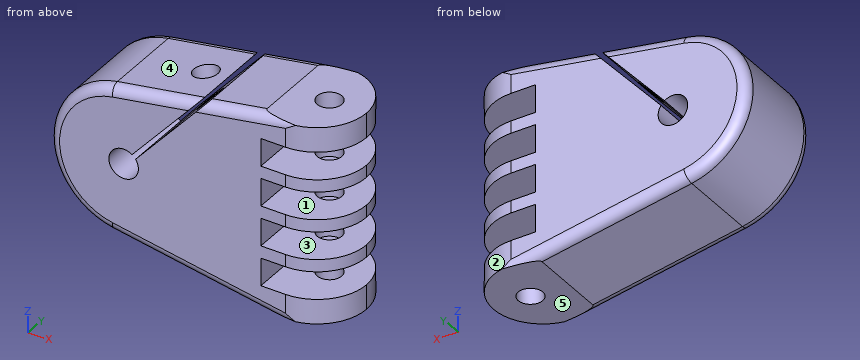
from build123d import *

# Parameters (mm, degrees)
BOSS_EXTRUDE1_DEPTH = 20
FILLET1_R           = 10
SKETCH2_R           = 2.5
CUT_EXTRUDE1_DEPTH  = 40
FILLET2_R           = 2
SKETCH3_R           = 2.5
CUT_EXTRUDE2_DEPTH  = 10
SKETCH4_R           = 10
SKETCH4_R_2         = 3
BOSS_EXTRUDE2_DEPTH = 20
CUT_EXTRUDE3_DEPTH  = 52.342938219


# Some blends are built 0.0001 mm under size
with BuildPart() as part:
    # Sketch1 → Boss-Extrude1 (new body)
    with BuildSketch(Plane(origin=(0, 0, 0), x_dir=(1, 0, 0), z_dir=(0, 1, 0))):
        with BuildLine():
            Line((27.849705815, 9.375), (27.849705815, 15))
            Line((27.849705815, 15), (42.849705815, 15))
            Line((42.849705815, 15), (42.849705815, 20))
            Line((42.849705815, 20), (27.849705815, 20))
            Line((27.849705815, 20), (-2.537743238, 14.78377013))
            ThreePointArc((-2.537743238, 14.78377013), (-15, 0), (-2.537743238, -14.78377013))
            Line((-2.537743238, -14.78377013), (15.176440556, -17.824540498))
            Line((15.176440556, -17.824540498), (6.327966589, -7.743180151))
            ThreePointArc((6.327966589, -7.743180151), (-6.707251498, 7.417059885), (7.069754095, -7.072381285))
            Line((7.069754095, -7.072381285), (16.743020962, -18.093455585))
            Line((16.743020962, -18.093455585), (27.849705815, -20))
            Line((27.849705815, -20), (42.849705815, -20))
            Line((42.849705815, -20), (42.849705815, -15))
            Line((42.849705815, -15), (27.849705815, -15))
            Line((27.849705815, -15), (27.849705815, -9.375))
            Line((27.849705815, -9.375), (42.849705815, -9.375))
            Line((42.849705815, -9.375), (42.849705815, -6.875))
            Line((42.849705815, -6.875), (27.849705815, -6.875))
            Line((27.849705815, -6.875), (27.849705815, -1.25))
            Line((27.849705815, -1.25), (42.849705815, -1.25))
            Line((42.849705815, -1.25), (42.849705815, 1.25))
            Line((42.849705815, 1.25), (27.849705815, 1.25))
            Line((27.849705815, 1.25), (27.849705815, 6.875))
            Line((27.849705815, 6.875), (42.849705815, 6.875))
            Line((42.849705815, 6.875), (42.849705815, 9.375))
            Line((42.849705815, 9.375), (27.849705815, 9.375))
        make_face()
    extrude(amount=BOSS_EXTRUDE1_DEPTH)

    # Fillet1
    fillet1_edges = [part.edges().sort_by_distance(p)[0] for p in [
        (42.849705815, 0, 17.5),
        (42.849705815, 0, 8.125),
        (42.849705815, 0, 0),
        (42.849705815, 0, -8.125),
        (42.849705815, 0, -17.5),
        (42.849705815, 20, -17.5),
        (42.849705815, 20, -8.125),
        (42.849705815, 20, 0),
        (42.849705815, 20, 8.125),
        (42.849705815, 20, 17.5),
    ]]
    fillet(fillet1_edges, radius=FILLET1_R - 0.0001)  # a hair under: the kernel refuses the full size

    # Sketch2 → Cut-Extrude1 (cut)
    with BuildSketch(Plane(origin=(0, 0, -20), x_dir=(-1, 0, 0), z_dir=(0, 0, -1))):
        with Locations((-35.349705815, 10)):
            Circle(SKETCH2_R)
    extrude(amount=-CUT_EXTRUDE1_DEPTH, mode=Mode.SUBTRACT)

    # Fillet2
    # the kernel refuses this fillet: 2 mm, written as the material it takes off along each edge
    with BuildSketch(Plane(origin=(39.676721919, 0, -22.03019459), x_dir=(0.16918288251037936, 0, 0.9855846753402162), z_dir=(-0.9855846753402161, 0, 0.16918288251037933))) as fillet2_piece_1:
        with BuildLine():
            CenterArc((FILLET2_R, FILLET2_R), FILLET2_R, 180, 90)
            Line((0, FILLET2_R), (-FILLET2_R * 0.02, FILLET2_R))
            Line((-FILLET2_R * 0.02, FILLET2_R), (-FILLET2_R * 0.02, -FILLET2_R * 0.02))
            Line((-FILLET2_R * 0.02, -FILLET2_R * 0.02), (FILLET2_R, -FILLET2_R * 0.02))
            Line((FILLET2_R, -FILLET2_R * 0.02), (FILLET2_R, 0))
        make_face()
    extrude(amount=42.831900914, mode=Mode.SUBTRACT)
    with BuildSketch(Plane(origin=(-2.537743238, 0, 14.78377013), x_dir=(0.16918288251037944, 0, -0.9855846753402161), z_dir=(0.9855846753402161, 0, 0.16918288251037944))) as fillet2_piece_2:
        with BuildLine():
            CenterArc((FILLET2_R, FILLET2_R), FILLET2_R, 180, 90)
            Line((0, FILLET2_R), (-FILLET2_R * 0.02, FILLET2_R))
            Line((-FILLET2_R * 0.02, FILLET2_R), (-FILLET2_R * 0.02, -FILLET2_R * 0.02))
            Line((-FILLET2_R * 0.02, -FILLET2_R * 0.02), (FILLET2_R, -FILLET2_R * 0.02))
            Line((FILLET2_R, -FILLET2_R * 0.02), (FILLET2_R, 0))
        make_face()
    extrude(amount=29.973274379, mode=Mode.SUBTRACT)
    with BuildSketch(Plane(origin=(39.676721919, 20, -22.03019459), x_dir=(0.16918288251037936, 0, 0.9855846753402162), z_dir=(-0.9855846753402161, 0, 0.16918288251037933))) as fillet2_piece_3:
        with BuildLine():
            CenterArc((FILLET2_R, -FILLET2_R), FILLET2_R, 90, 90)
            Line((0, -FILLET2_R), (-FILLET2_R * 0.02, -FILLET2_R))
            Line((-FILLET2_R * 0.02, -FILLET2_R), (-FILLET2_R * 0.02, FILLET2_R * 0.02))
            Line((-FILLET2_R * 0.02, FILLET2_R * 0.02), (FILLET2_R, FILLET2_R * 0.02))
            Line((FILLET2_R, FILLET2_R * 0.02), (FILLET2_R, 0))
        make_face()
    extrude(amount=42.831900914, mode=Mode.SUBTRACT)
    with BuildSketch(Plane(origin=(-2.537743238, 20, 14.78377013), x_dir=(0.16918288251037944, 0, -0.9855846753402161), z_dir=(0.9855846753402161, 0, 0.16918288251037944))) as fillet2_piece_4:
        with BuildLine():
            CenterArc((FILLET2_R, -FILLET2_R), FILLET2_R, 90, 90)
            Line((0, -FILLET2_R), (-FILLET2_R * 0.02, -FILLET2_R))
            Line((-FILLET2_R * 0.02, -FILLET2_R), (-FILLET2_R * 0.02, FILLET2_R * 0.02))
            Line((-FILLET2_R * 0.02, FILLET2_R * 0.02), (FILLET2_R, FILLET2_R * 0.02))
            Line((FILLET2_R, FILLET2_R * 0.02), (FILLET2_R, 0))
        make_face()
    extrude(amount=29.973274379, mode=Mode.SUBTRACT)
    with BuildSketch(Plane(origin=(4.916004858, 0, 16.063260995), x_dir=(0.16918288251037944, 0, -0.9855846753402161), z_dir=(0.9855846753402161, 0, 0.16918288251037944))) as fillet2_piece_5:
        with BuildLine():
            CenterArc((FILLET2_R, FILLET2_R), FILLET2_R, 180, 90)
            Line((0, FILLET2_R), (-FILLET2_R * 0.02, FILLET2_R))
            Line((-FILLET2_R * 0.02, FILLET2_R), (-FILLET2_R * 0.02, -FILLET2_R * 0.02))
            Line((-FILLET2_R * 0.02, -FILLET2_R * 0.02), (FILLET2_R, -FILLET2_R * 0.02))
            Line((FILLET2_R, -FILLET2_R * 0.02), (FILLET2_R, 0))
        make_face()
    extrude(amount=35.269133064, mode=Mode.SUBTRACT)
    with BuildSketch(Plane(origin=(4.916004858, 20, 16.063260995), x_dir=(0.16918288251037944, 0, -0.9855846753402161), z_dir=(0.9855846753402161, 0, 0.16918288251037944))) as fillet2_piece_6:
        with BuildLine():
            CenterArc((FILLET2_R, -FILLET2_R), FILLET2_R, 90, 90)
            Line((0, -FILLET2_R), (-FILLET2_R * 0.02, -FILLET2_R))
            Line((-FILLET2_R * 0.02, -FILLET2_R), (-FILLET2_R * 0.02, FILLET2_R * 0.02))
            Line((-FILLET2_R * 0.02, FILLET2_R * 0.02), (FILLET2_R, FILLET2_R * 0.02))
            Line((FILLET2_R, FILLET2_R * 0.02), (FILLET2_R, 0))
        make_face()
    extrude(amount=35.269133064, mode=Mode.SUBTRACT)
    with BuildSketch(Plane(origin=(0, 0, 0), x_dir=(-0.16918288251037905, 0, -0.9855846753402162), z_dir=(0.9855846753402162, 0, -0.16918288251037905))) as fillet2_piece_7:
        with BuildLine():
            CenterArc((15 - FILLET2_R, FILLET2_R), FILLET2_R, 270, 90)
            Line((15, FILLET2_R), (15 + FILLET2_R * 0.02, FILLET2_R))
            Line((15 + FILLET2_R * 0.02, FILLET2_R), (15 + FILLET2_R * 0.02, -FILLET2_R * 0.02))
            Line((15 + FILLET2_R * 0.02, -FILLET2_R * 0.02), (15 - FILLET2_R, -FILLET2_R * 0.02))
            Line((15 - FILLET2_R, -FILLET2_R * 0.02), (15 - FILLET2_R, 0))
        make_face()
    revolve(axis=Axis((0, 0, 0), (0, 1, 0)), revolution_arc=160.519372943, mode=Mode.SUBTRACT)
    with BuildSketch(Plane(origin=(0, 20, 0), x_dir=(-0.16918288251037905, 0, -0.9855846753402162), z_dir=(0.9855846753402162, 0, -0.16918288251037905))) as fillet2_piece_8:
        with BuildLine():
            CenterArc((15 - FILLET2_R, -FILLET2_R), FILLET2_R, 0, 90)
            Line((15, -FILLET2_R), (15 + FILLET2_R * 0.02, -FILLET2_R))
            Line((15 + FILLET2_R * 0.02, -FILLET2_R), (15 + FILLET2_R * 0.02, FILLET2_R * 0.02))
            Line((15 + FILLET2_R * 0.02, FILLET2_R * 0.02), (15 - FILLET2_R, FILLET2_R * 0.02))
            Line((15 - FILLET2_R, FILLET2_R * 0.02), (15 - FILLET2_R, 0))
        make_face()
    revolve(axis=Axis((0, 20, 0), (0, 1, 0)), revolution_arc=160.519372943, mode=Mode.SUBTRACT)

    # Sketch3 → Cut-Extrude2 (cut)
    with BuildSketch(Plane(origin=(-2.537743238, 0, 14.78377013), x_dir=(0.9855846753402161, 0, 0.16918288251037955), z_dir=(-0.16918288251037955, 0, 0.9855846753402161))):
        with Locations((12.973274379, 10)):
            Circle(SKETCH3_R)
    extrude(amount=-CUT_EXTRUDE2_DEPTH, mode=Mode.SUBTRACT)

    # Sketch4 → Boss-Extrude2 (add)
    with BuildSketch(Plane.XZ):
        Circle(SKETCH4_R)
        with Locations(Location((0, 0, 0), (0, 0, 270))):
            Circle(SKETCH4_R_2, mode=Mode.SUBTRACT)
    extrude(amount=-BOSS_EXTRUDE2_DEPTH)

    # Sketch6 → Cut-Extrude3 (cut, through all)
    with BuildSketch(Plane.XZ):
        with BuildLine():
            ThreePointArc((7.069754095, 7.072381285), (6.707251498, 7.417059885), (6.327966589, 7.743180151))
            Line((6.327966589, 7.743180151), (1.700797535, 2.471292727))
            ThreePointArc((1.700797535, 2.471292727), (2.089347904, 2.152817999), (2.419304242, 1.773969274))
            Line((2.419304242, 1.773969274), (7.069754095, 7.072381285))
        make_face()
    extrude(amount=-CUT_EXTRUDE3_DEPTH, mode=Mode.SUBTRACT)


solid = part.part
Build history of the part. All positions in model axes, mm. Face numbers are marked on the shaded views. A direction names the side the tool comes from. Coordinates: 2 decimals unless noted, no trailing zeros. Write each loop counter-clockwise with the first axis right and the second up, starting at its lowest first coordinate (ties: lowest second). Pieces come first, ordered by that corner, then holes. Notation, with made-up numbers: (-35, 89) -> (23, 89) arc R10 ccw to (23, 98) -> close; hole circle Ø7 at (32.25, 51). An arc over 180 degrees is marked (long way). Use CSV: the item, a comma, the result in double quotes. Start each with the question number.
Q1. Pull direction Z, two halves, no side cores. Call the marked faces 3, 4 and 5: released by +Z, released by -Z, zero draft, split by the parting line, or undercut.
Q2. 3-axis set-ups, long thin cutter, end or side, ignore diameter. For the marked faces 1 and 2: which of +Z, -Z, +X, -X, +Y, -Y reach the whole face in a straight line?
Q3. Cut at A-A, the plane z = 0. State how many separate pieces and enclosed holes the cut face has, then the cut area to 3 significant figures.
Q4. Cut at C-C, the plane y = 3. List the corners of the cut face in (x, z) (3 decimals), then the cut area to 3 significant figures.
Q5. Flat gauge pins, fed straight in: pin 1 Ø6.5 at (x, y) = (35.35, 10) entering from +Z; pin 2 Ø10 at (y, z) = (8.5, 7.5) entering from -X; pin 3 Ø4.5 at (y, z) = (5.5, 13) entering from +X; pin 4 Ø1 at (y, z) = (14.5, 6.5) entering from -X. Where does each tip first touch, or does it go through?
Q6. Drill centre lines: probe 1 along Z at (x, y) = (39.5, 12.75) (3 decimals); probe 2 along X at (y, z) = (10.5, 0); probe 3 along X at (y, z) = (9.5, 8). Where is each one in solid material? Low to high.
Checked values:
1,face 3,"undercut"
1,face 4,"released by +Z"
1,face 5,"released by -Z"
2,face 1,"+X, +Y, -Y"
2,face 2,"+Z, -Z, +X, +Y"
3,separate pieces,"2"
3,enclosed holes,"1"
3,area,"973 mm²"
4,outline,"(-2.538, -14.784) -> (27.85, -20) -> (39.991, -20) -> (39.991, -15) -> (27.85, -15) -> (27.85, -9.375) -> (39.991, -9.375) -> (39.991, -6.875) -> (27.85, -6.875) -> (27.85, -1.25) -> (39.991, -1.25) -> (39.991, 1.25) -> (27.85, 1.25) -> (27.85, 6.875) -> (39.991, 6.875) -> (39.991, 9.375) -> (27.85, 9.375) -> (27.85, 15) -> (39.991, 15) -> (39.991, 20) -> (27.85, 20) -> (16.743, 18.093) -> (2.419, 1.774) arc R3 cw (long way) to (1.701, 2.471) -> (15.176, 17.825) -> (-2.538, 14.784) arc R15 ccw to start"
4,area,"1,500 mm²"
5,pin 1,"stops at z = 20"
5,pin 2,"stops at x = -14.79"
5,pin 3,"stops at x = 42.23"
5,pin 4,"stops at x = -13.75"
6,probe 1,"z = -20 to -15, -9.375 to -6.875, -1.25 to 1.25, 6.875 to 9.375, 15 to 20"
6,probe 2,"x = -15 to -3, 3 to 32.9, 37.8 to 42.84"
6,probe 3,"x = -12.69 to 6.55, 7.88 to 9.3, 14.28 to 32.9, 37.8 to 42.84"
